For this review, use the dimensioned drawing (mm, ordinates from the lowest corner) and the shaded views. A direction names the side the tool comes from. Give positions to 0.01 mm unless a question says otherwise; leave off trailing zeros. Loops run counter-clockwise (first coordinate to the right, second up) from the corner with the lowest first, then second, coordinate; pieces in that order, holes last. Notation, with made-up numbers: (-37.5, 17.25) -> (-29.5, 17.25) arc R14 ccw to (-29.5, 26.25) -> close; hole circle Ø5 at (-4, 76). An arc over 180 degrees is marked (long way). Write each question's results on one line, items separated by ' | '. Start each with the question number.
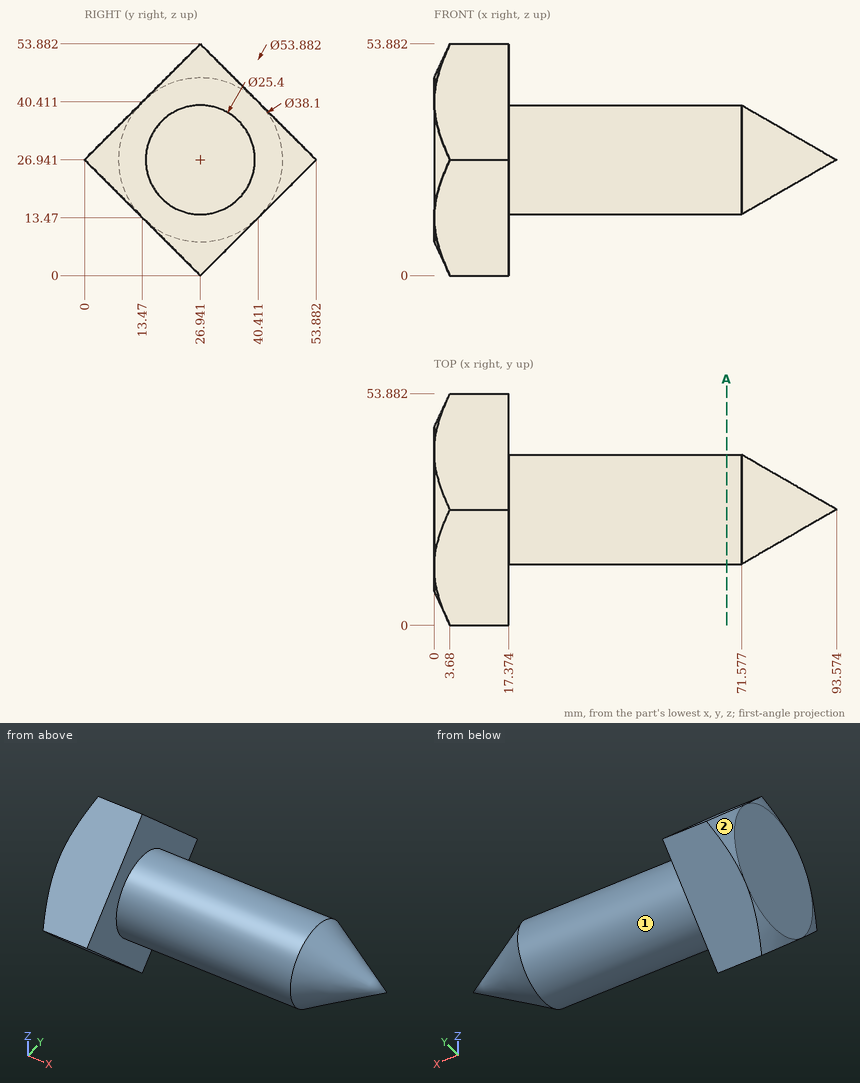
1. For pin 1 Ø12 at (y, z) = (44, 6.5) entering from -X; pin 2 Ø6 at (x, z) = (71.5, 19.5) entering from +Y; pin 3 Ø4 at (x, z) = (56, 14) entering from -Y; pin 4 Ø10 at (x, y) = (12, 29.5) entering from +Z, all flat-tipped, find the tip position at first contact; note any pin that passes through.
2. Machinability: for the marked faces 1 and 2, which of the approach directions +Z, -Z, +X, -X, +Y, -Y give a long, thin tool a straight path to every point of the face, cutting with its end or side? Answer none if there is none.
3. Wall thickness on L1, parallel to X at y = 45, z = 29; L2, parallel to Z at x = 68, y = 27; L3, parallel to Z at x = 5.5, y = 48 (1 decimal): over which ranges is each line inside the solid? List them lowest first.
4. We need section A-A (x = 68). Write out the cut boundary in (y, z), plus the area to 3 significant figures.
Response:
1) pin 1: passes through | pin 2: stops at y = 38.84 | pin 3: stops at y = 20.49 | pin 4: stops at z = 53.88
2) face 1: +X | face 2: -X, +Y
3) L1: x = 0 to 17.37 | L2: z = 14.24 to 39.64 | L3: z = 21.1 to 32.8
4) outline: circle Ø25.4 at (26.94, 26.94) | area: 507 mm2
